The drawing under review shows one solid part. Ordinate dimensions are in mm from its lowest x, y, z. A direction names the side the tool comes from. Give positions to 0.01 mm unless a question says otherwise; leave off trailing zeros. Loops run counter-clockwise (first coordinate to the right, second up) from the corner with the lowest first, then second, coordinate; pieces in that order, holes last.
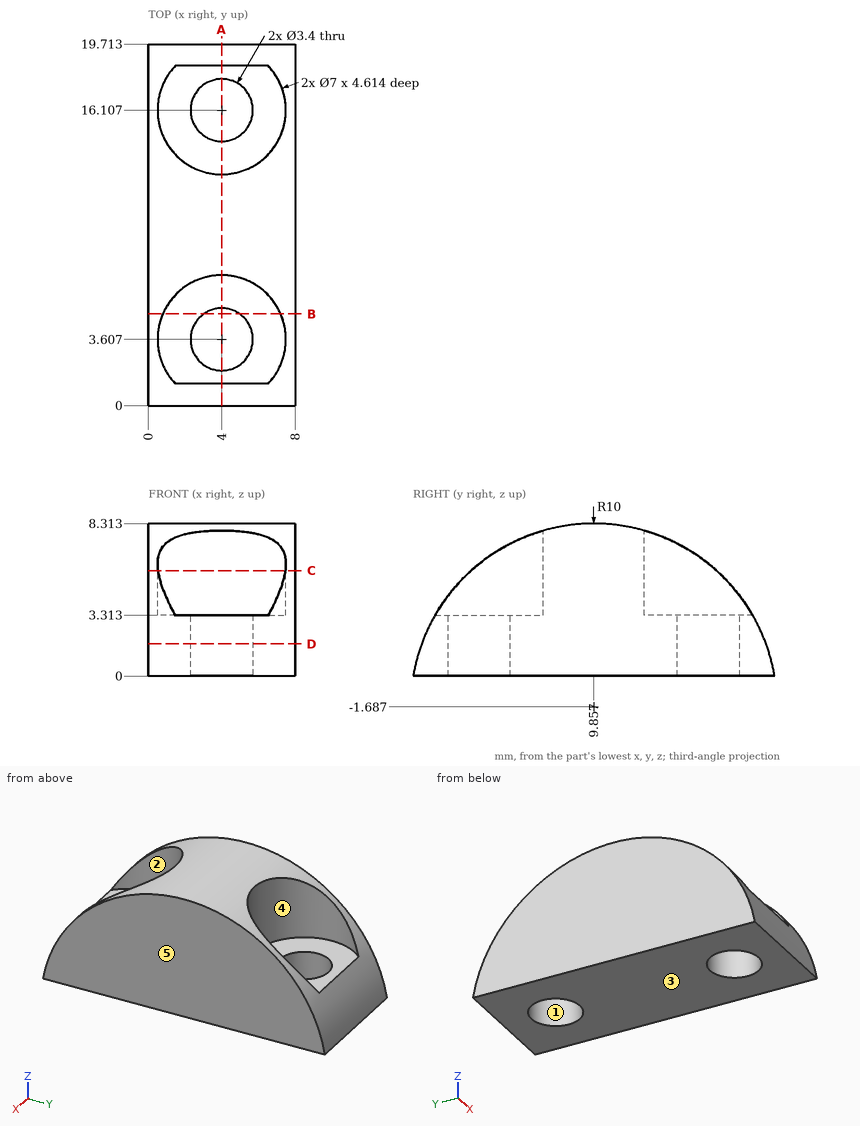
Item 1: For L1, parallel to Y at x = 3.75, z = 3 (1 decimal); L2, parallel to Y at x = 4, z = 2.5 (1 decimal); L3, parallel to X at y = 3.5, z = 0.5, list the stretches that pass through material, from the lowest coordinate up.
Answer:
L1: y = 1 to 1.9, 5.3 to 14.4, 17.8 to 18.7
L2: y = 0.8 to 1.9, 5.3 to 14.4, 17.8 to 18.9
L3: x = 0 to 2.3, 5.7 to 8
Item 2: Take a section at B-B on y = 5. Give the boundary of the cut face in (x, z).
Answer:
outline: (0, 0) - (3.03, 0) - (3.03, 3.31) - (0.79, 3.31) - (0.79, 7.05) - (0, 7.05) - close; (4.97, 0) - (8, 0) - (8, 7.05) - (7.21, 7.05) - (7.21, 3.31) - (4.97, 3.31) - close
Item 3: Take a section at C-C on z = 5.75. Give the boundary of the cut face in (x, y), and give its area (3 significant figures).
Answer:
outline: (0, 3.17) - (0.53, 3.17) arc R3.5 cw (long way) to (7.47, 3.17) - (8, 3.17) - (8, 16.54) - (7.47, 16.54) arc R3.5 cw (long way) to (0.53, 16.54) - (0, 16.54) - close
area: 62.4 mm2
Item 4: Tool access review of the marked faces 1 and 2: name each direction out of +Z, -Z, +X, -X, +Y, -Y from which nothing blocks a thin tool from reaching the whole face with its end or side.
Answer:
face 1: +Z, -Z
face 2: +Z
Item 5: Clearance check with flat-ended pins moving along their axes: pin 1 Ø4 at (x, y) = (4, 16.11) entering from +Z; pin 2 Ø1.5 at (x, y) = (1, 12.5) entering from +Z; pin 3 Ø2 at (x, z) = (3, 6) entering from -Y; pin 4 Ø3 at (x, z) = (2.5, 1.5) entering from -Y. State where each tip first meets the part, or that it passes through.
Answer:
pin 1: stops at z = 3.31
pin 2: stops at z = 8.13
pin 3: stops at y = 6.48
pin 4: stops at y = 0
Item 6: The part is to be moulded in two halves that separate along X. For the marked faces 3, 4 and 5, say which applies: released by +X, released by -X, zero draft, split by the parting line, or undercut.
Answer:
face 3: zero draft
face 4: undercut
face 5: released by +X
Item 7: Take a section at D-D on z = 1.75. Give the boundary of the cut face in (x, y), and give its area (3 significant figures).
Answer:
outline: (0, 0.47) - (8, 0.47) - (8, 19.25) - (0, 19.25) - close; hole circle Ø3.4 at (4, 3.61); hole circle Ø3.4 at (4, 16.11)
area: 132 mm2
Item 8: Take a section at A-A on x = 4. Give the boundary of the cut face in (y, z).
Answer:
outline: (0, 0) - (1.91, 0) - (1.91, 3.31) - (1.2, 3.31) arc R10 ccw to start; (5.31, 0) - (14.41, 0) - (14.41, 3.31) - (12.61, 3.31) - (12.61, 7.93) arc R10 ccw to (7.11, 7.93) - (7.11, 3.31) - (5.31, 3.31) - close; (17.81, 0) - (19.71, 0) arc R10 ccw to (18.52, 3.31) - (17.81, 3.31) - close
